```python
from build123d import *

# Parameters (mm, degrees)
SCHIZZO1_R                   = 3.3095
ESTRUSIONE_ESTRUSIONE1_DEPTH = 8
RACCORDO1_R                  = 0.48
SMUSSO1_SIZE                 = 0.6905


with BuildPart() as part:
    # Schizzo1 → Estrusione-Estrusione1 (new body)
    with BuildSketch(Plane.XY):
        Polygon((0, 7.505553499), (-6.5, 3.75277675), (-6.5, -3.75277675), (0, -7.505553499), (6.5, -3.75277675), (6.5, 3.75277675), align=None)
        Circle(SCHIZZO1_R, mode=Mode.SUBTRACT)
    extrude(amount=ESTRUSIONE_ESTRUSIONE1_DEPTH)

    # Schizzo2 → Rivoluzione1 (revolve)
    with BuildSketch(Plane(origin=(0, 0, 0), x_dir=(0, 0, -1), z_dir=(1, 0, 0)), mode=Mode.PRIVATE) as rivoluzione1_sk:
        with BuildLine():
            Line((0, 3.3095), (0, 8.331345278))
            ThreePointArc((0, 8.331345278), (-0.511226457, 8.940601245), (-1.2, 8.542937654))
            Line((-1.2, 8.542937654), (-3.104815529, 3.3095))
            Line((-3.104815529, 3.3095), (0, 3.3095))
        make_face()
    revolve(rivoluzione1_sk.sketch.rotate(Axis((0, 0, 0), (0, 0, 1)), 90), axis=Axis((0, 0, 0), (0, 0, 1)))

    # Schizzo3 → Taglia-Rivoluzione1 (revolve, cut)
    with BuildSketch(Plane(origin=(0, 0, 0), x_dir=(0, 0, -1), z_dir=(1, 0, 0)), mode=Mode.PRIVATE) as taglia_rivoluzione1_sk:
        Polygon((-8, 6.5), (-7.2, 7.505553499), (-7.2, 20.205553499), (-20.7, 20.205553499), (-20.7, 6.5), align=None)
    revolve(taglia_rivoluzione1_sk.sketch.rotate(Axis((0, 0, 8), (0, 0, -1)), 270), axis=Axis((0, 0, 8), (0, 0, -1)), mode=Mode.SUBTRACT)

    # Raccordo1
    raccordo1_edges = [part.edges().sort_by_distance(p)[0] for p in [
        (-6.5, -1.884573791, 1.846137562),
        (-3.25, -5.629165125, 1.943568497),
        (3.25, -5.629165125, 1.943568497),
        (6.5, 0, 1.943568497),
        (3.25, 5.629165125, 1.943568497),
        (-3.25, 5.629165125, 1.943568497),
        (-6.5, 1.884573791, 1.846137562),
    ]]
    fillet(raccordo1_edges, radius=RACCORDO1_R)

    # Smusso1
    smusso1_edges = [part.edges().sort_by_distance(p)[0] for p in [
        (-3.3095, 0, 0),
        (-3.3095, 0, 8),
    ]]
    chamfer(smusso1_edges, length=SMUSSO1_SIZE)


solid = part.part
```
Can you work these out from the model? Positions are in its coordinate system, mm. A direction names the side the tool comes from. Coordinates: 2 decimals unless noted, no trailing zeros. Write each loop counter-clockwise with the first axis right and the second up, starting at its lowest first coordinate (ties: lowest second). Pieces come first, ordered by that corner, then holes. Notation, with made-up numbers: M 57.5,-19 L 108.5,-19 A12 ccw 108.5,1 Z; hole C 50.25,5 d8. An arc over 180 degrees is marked long. Write item = value, one per line. Start each with the question number.
Q1. If we section it at A-A, the plane z = 4.5: Write out the boundary of the cut face in (x, y).
Q2. I'm going to push flat-ended pins straight in: pin 1 (3 mm diameter, centred on y = 2, z = 4, fed in from +X); pin 2 (8.5 mm diameter, centred on x = 0, y = 0, fed in from -Z); pin 3 (1 mm diameter, centred on x = 0, z = 6, fed in from -Y); pin 4 (3 mm diameter, centred on x = 7, z = 6.5, fed in from +Y). Where does each tip first touch, or does it pass through?
Q3. On a 3-axis mill with a long thin cutter (end or side, diameter ignored), from which of +Z, -Z, +X, -X, +Y, -Y can I reach the whole of each face in a straight line? I mean faces 4 (the face through (-3.2, 5.66, 4.93)), 5 (the face through (0.02, -6.74, 7.81)), 6 (the face through (3.3, 5.6, 4.9)), 7 (the face through (3.2, -5.66, 4.93)), 8 (the face through (-3.3, -5.6, 4.9)). Say none if no direction works.
Q4. Thinking about a two-plate mould opening in Y: for faces 1 (the face through (5.833, 3.386, 7.806)), 2 (the face through (-0.72, -3.23, 3.95)), 3 (the face through (-6.5, 0, 5)), which applies, released by +Y, released by -Y, zero draft, split by the parting line, or undercut?
Q5. If I drill on L1, parallel to X at y = 2.25, z = 3; L2, parallel to Y at x = -1, z = 1; L3, parallel to Y at x = -0.75, z = 3.5, over which ranges is the centre line in solid material (lowest first)? Write a range as [from, to].
Check sheet entries:
q1.outline = M -6.5,-3.75 L 0,-7.51 L 6.5,-3.75 L 6.5,3.75 L 0,7.51 L -6.5,3.75 Z; hole C 0,0 d6.62
q2.pin_1 = 6.5
q2.pin_2 = 0
q2.pin_3 = -7.51
q2.pin_4 = 4.33
q3.face_4 = +Z, -X, +Y
q3.face_5 = +Z, -Y
q3.face_6 = +Z, +X, +Y
q3.face_7 = +Z, +X, -Y
q3.face_8 = +Z, -X, -Y
q4.face_1 = released by +Y
q4.face_2 = undercut
q4.face_3 = zero draft
q5.L1 = [-6.5, -2.43], [2.43, 6.5]
q5.L2 = [-8.76, -3.15], [3.15, 8.76]
q5.L3 = [-7.07, -3.22], [3.22, 7.07]
